Input: part model. Units: mm. Frame: model coordinates. A direction names the side the tool comes from. Give positions to 0.01 mm unless a question says otherwise; leave off trailing zeros. Loops run counter-clockwise (first coordinate to the right, second up) from the corner with the lowest first, then second, coordinate; pieces in that order, holes last.
from build123d import *

# Parameters (mm, degrees)
SKETCH1_R           = 1.27
BOSS_EXTRUDE1_DEPTH = 3.175


with BuildPart() as part:
    # Sketch1 → Boss-Extrude1 (new body)
    with BuildSketch(Plane.XY):
        with BuildLine():
            Line((-19.353012887, 0), (-19.353012887, 68.58))
            ThreePointArc((-19.353012887, 68.58), (-20.096961663, 70.376051224), (-21.893012887, 71.12))
            Line((-21.893012887, 71.12), (-35.863012887, 71.12))
            ThreePointArc((-35.863012887, 71.12), (-37.659064112, 71.863948776), (-38.403012887, 73.66))
            Line((-38.403012887, 73.66), (-38.403012887, 81.28))
            ThreePointArc((-38.403012887, 81.28), (-37.659064112, 83.076051224), (-35.863012887, 83.82))
            Line((-35.863012887, 83.82), (16.206987113, 83.82))
            ThreePointArc((16.206987113, 83.82), (18.003038337, 83.076051224), (18.746987113, 81.28))
            Line((18.746987113, 81.28), (18.746987113, 73.66))
            ThreePointArc((18.746987113, 73.66), (18.003038337, 71.863948776), (16.206987113, 71.12))
            Line((16.206987113, 71.12), (2.236987113, 71.12))
            ThreePointArc((2.236987113, 71.12), (0.440935888, 70.376051224), (-0.303012887, 68.58))
            Line((-0.303012887, 68.58), (-0.303012887, 0))
            ThreePointArc((-0.303012887, 0), (-9.828012887, -9.525), (-19.353012887, 0))
        make_face()
        with Locations((-9.828012887, 0)):
            Circle(SKETCH1_R, mode=Mode.SUBTRACT)
    extrude(amount=BOSS_EXTRUDE1_DEPTH)


solid = part.part
(1) Cut plane B-B (y = 11). Return the cut outline in (x, z) (3 decimals).
Values follow:
outline: (-19.353, 0) - (-0.303, 0) - (-0.303, 3.175) - (-19.353, 3.175) - close
(2) Cut plane C-C (x = -32.5). Return the cut outline in (y, z) (3 decimals), and give its area (3 significant figures).
Values follow:
outline: (71.12, 0) - (83.82, 0) - (83.82, 3.175) - (71.12, 3.175) - close
area: 40.3 mm2
(3) Ray query, probe 1 along X at (y, z) = (23, 1.3); probe 2 along Y at (x, z) = (15, 1.3); probe 3 along Y at (x, z) = (-13.5, 1.15). Return the intervals inside material, ascending.
Values follow:
probe 1: x = -19.35 to -0.3
probe 2: y = 71.12 to 83.82
probe 3: y = -8.79 to 83.82
(4) Pin query (flat end, axial travel): pin 1 Ø1 at (y, z) = (46, 1.5) entering from -X; pin 2 Ø1.5 at (x, z) = (-1, 2) entering from -Y; pin 3 Ø1 at (x, z) = (12, 1) entering from -Y. Return the tip coordinate at first contact, or that it passes through.
Values follow:
pin 1: stops at x = -19.35
pin 2: stops at y = -5.05
pin 3: stops at y = 71.12
(5) Reachability of faces 5 (the flat face through (-10, 83.82, 2)), 6 (the flat face through (9, 71.12, 2)) from +Z, -Z, +X, -X, +Y, -Y: full face, straight path, thin tool, end or side. Return the list, or none.
Values follow:
face 5: +Z, -Z, +X, -X, +Y
face 6: +Z, -Z, +X, -Y
(6) Mould query, pull axis X, two halves, no side actions, for faces 1 (the flat face through (-29, 71.12, 2)), 2 (the cylindrical face through (17.98, 83.1, 1.57)), 3 (the flat face through (-19.353, 34, 2)), 4 (the cylindrical face through (-8.655, -0.486, 1.565)). Classes: +X half, -X half, draft (parallel to the pull), parting line (faces both ways), or undercut.
Values follow:
face 1: draft
face 2: +X half
face 3: -X half
face 4: undercut
(7) Cut plane A-A (z = 1.9). Return the cut outline in (x, y) (3 decimals), and give its area (3 significant figures).
Values follow:
outline: (-38.403, 73.66) arc R2.54 ccw to (-35.863, 71.12) - (-21.893, 71.12) arc R2.54 cw to (-19.353, 68.58) - (-19.353, 0) arc R9.525 ccw to (-0.303, 0) - (-0.303, 68.58) arc R2.54 cw to (2.237, 71.12) - (16.207, 71.12) arc R2.54 ccw to (18.747, 73.66) - (18.747, 81.28) arc R2.54 ccw to (16.207, 83.82) - (-35.863, 83.82) arc R2.54 ccw to (-38.403, 81.28) - close; hole circle Ø2.54 at (-9.828, 0)
area: 2,220 mm2
